Geometry: final body of the model. Coordinates: model frame, mm. A direction names the side the tool comes from. Round coordinates to 2 decimals unless told otherwise and drop trailing zeros. Loops run counter-clockwise (first coordinate to the right, second up) from the corner with the lowest first, then second, coordinate; pieces in that order, holes last. Notation, with made-up numbers: M 1.25,-10 L 57.25,-10 A35 cw 57.25,23 Z; hole C 42.5,48.25 d9. An arc over 180 degrees is marked long. Answer as a JSON object with one key per item and string values.
from build123d import *

# Parameters (mm, degrees)
F0_W      = 30
F0_H      = 32
F1_DEPTH  = 0.2
F2_W      = 30
F2_H      = 32
F2_W_2    = 28
F2_H_2    = 30
F3_DEPTH  = 1.4
F4_W      = 28
F4_H      = 20
F5_DEPTH  = 0.2
F6_W      = 28
F6_H      = 10
F7_DEPTH  = 0.2
F3_FACE_W = 32
F3_FACE_H = 1.6
F8_DEPTH  = 10
F9_W      = 11
F9_H      = 16
F10_DEPTH = 1.4


with BuildPart() as f1:
    # F0 (on Top) → F1 (new body)
    with BuildSketch(Plane.XY):
        with Locations((15, -16)):
            Rectangle(F0_W, F0_H)
    extrude(amount=F1_DEPTH)

    # F2 (on face) → F3 (join)
    with BuildSketch(Plane.XY.offset(0.2)):
        with Locations((15, -16)):
            Rectangle(F2_W, F2_H)
        with Locations((15, -16)):
            Rectangle(F2_W_2, F2_H_2, mode=Mode.SUBTRACT)
    extrude(amount=F3_DEPTH)

    # F4 (on face) → F5 (join)
    with BuildSketch(Plane.XY.offset(0.2)):
        with Locations((15, -11)):
            Rectangle(F4_W, F4_H)
    extrude(amount=F5_DEPTH)

    # F6 (on face) → F7 (join)
    with BuildSketch(Plane.XY.offset(0.4)):
        with Locations((15, -6)):
            Rectangle(F6_W, F6_H)
    extrude(amount=F7_DEPTH)

    # F3_face (on face) → F8 (join)
    with BuildSketch(Plane(origin=(30, -16, 0.8), x_dir=(0, 1, 0), z_dir=(1, 0, 0))):
        Rectangle(F3_FACE_W, F3_FACE_H)
    extrude(amount=F8_DEPTH)

    # F9 (on face) → F10 (join)
    with BuildSketch(Plane.XY.offset(1.6)):
        with Locations((34.5, -8)):
            Rectangle(F9_W, F9_H)
    extrude(amount=F10_DEPTH)


solid = f1.part
1) Section query C-C (y = -25). Return the cut outline in (x, z), and give its area (3 significant figures).
Results:
{"outline": "M 0,0 L 40,0 L 40,1.6 L 29,1.6 L 29,0.2 L 1,0.2 L 1,1.6 L 0,1.6 Z", "area": "24.8 mm2"}
2) Section query B-B (x = 17). Return the cut outline in (y, z).
Results:
{"outline": "M -32,0 L 0,0 L 0,1.6 L -1,1.6 L -1,0.6 L -11,0.6 L -11,0.4 L -21,0.4 L -21,0.2 L -31,0.2 L -31,1.6 L -32,1.6 Z"}
3) Pull-direction query (Y, two-part tool) for faces 6 (the flat face through (24, 0, 1)), 7 (the flat face through (20, -32, 1)), 8 (the flat face through (15, -1, 1)); classes: +Y half, -Y half, draft (parallel to the pull), parting line (faces both ways), or undercut.
Results:
{"face 6": "+Y half", "face 7": "-Y half", "face 8": "undercut"}
4) Pin query (flat end, axial travel): P1, Ø3, axis at x = 13, y = -28.5, coming from the +Z side; P2, Ø5, axis at x = 20.5, y = -15.5, coming from the +Z side; P3, Ø1.5, axis at x = 30, y = -28, coming from the +Z side. Return the tip coordinate at first contact, or that it passes through.
Results:
{"P1": "z = 0.2", "P2": "z = 0.4", "P3": "z = 1.6"}
5) Section query A-A (z = 1.15). Return the cut outline in (x, y).
Results:
{"outline": "M 0,-32 L 40,-32 L 40,0 L 0,0 Z; hole M 1,-31 L 29,-31 L 29,-1 L 1,-1 Z"}
6) Reachability of faces 1 (the flat face through (0, -16, 1)), 2 (the flat face through (40, -13, 1)), 3 (the flat face through (30, -20, 1.6)), 4 (the flat face through (15, -6, 0.6)), 5 (the flat face through (34, -16, 2)) from +Z, -Z, +X, -X, +Y, -Y: full face, straight path, thin tool, end or side. Return the list, or none.
Results:
{"face 1": "+Z, -Z, -X, +Y, -Y", "face 2": "+Z, -Z, +X, +Y, -Y", "face 3": "+Z, -X, -Y", "face 4": "+Z", "face 5": "+Z, +X, -X, -Y"}
7) Ray query, line 1 (Y direction, x = 11, z = 0.5); line 2 (Y direction, x = 19.5, z = 0.25); line 3 (X direction, y = -23, z = 1.45). Return the intervals inside material, ascending.
Results:
{"line 1": "-32 to -31, -11 to 0", "line 2": "-32 to -31, -21 to 0", "line 3": "0 to 1, 29 to 40"}
8) Section query D-D (y = -15.5). Return the cut outline in (x, z).
Results:
{"outline": "M 0,0 L 40,0 L 40,3 L 29,3 L 29,0.4 L 1,0.4 L 1,1.6 L 0,1.6 Z"}
